from build123d import *

# Parameters (mm, degrees)
SKETCH1_R           = 11.495405
BOSS_EXTRUDE2_DEPTH = 4.7625
BOSS_EXTRUDE3_DEPTH = 3.175
FILLET1_R           = 1.5875


with BuildPart() as part:
    # Sketch1 → Boss-Extrude2 (new body, symmetric)
    with BuildSketch(Plane.XY):
        with BuildLine():
            ThreePointArc((14.672983865, 0.491098707), (-4.158599684, 14.079903484), (-12.585193267, -7.559797873))
            ThreePointArc((-12.585193267, -7.559797873), (4.158599684, -14.079903484), (14.672983865, 0.491098707))
        make_face()
        Circle(SKETCH1_R, mode=Mode.SUBTRACT)
    extrude(amount=BOSS_EXTRUDE2_DEPTH, both=True)

    # Sketch1<4> → Boss-Extrude3 (add, symmetric)
    with BuildSketch(Plane.XY):
        with BuildLine():
            ThreePointArc((-12.585193267, -7.559797873), (-10.89585042, -11.492870345), (-10.31875, -15.734319794))
            Line((-10.31875, -15.734319794), (-10.31875, -56.374319794))
            Line((-10.31875, -56.374319794), (8.54075, -56.374319794))
            Line((8.54075, -56.374319794), (8.54075, -76.694319794))
            Line((8.54075, -76.694319794), (34.499171822, -69.027315193))
            Line((34.499171822, -69.027315193), (23.458960581, -51.968120144))
            Line((23.458960581, -51.968120144), (39.292025986, -41.721424085))
            Line((39.292025986, -41.721424085), (17.211603503, -7.603033986))
            ThreePointArc((17.211603503, -7.603033986), (15.391641433, -3.728672569), (14.672983865, 0.491098707))
            ThreePointArc((14.672983865, 0.491098707), (4.158599684, -14.079903484), (-12.585193267, -7.559797873))
        make_face()
        with BuildLine():
            ThreePointArc((5.55625, -46.055569794), (0, -51.611819794), (-5.55625, -46.055569794))
            Line((-5.55625, -46.055569794), (-5.55625, -34.943069794))
            ThreePointArc((-5.55625, -34.943069794), (0, -29.386819794), (5.55625, -34.943069794))
            Line((5.55625, -34.943069794), (5.55625, -46.055569794))
        make_face(mode=Mode.SUBTRACT)
        with BuildLine():
            ThreePointArc((29.687419875, -35.646101109), (28.04160399, -43.329532516), (20.358172583, -41.683716631))
            Line((20.358172583, -41.683716631), (14.32055706, -32.354469339))
            ThreePointArc((14.32055706, -32.354469339), (15.966372945, -24.671037931), (23.649804353, -26.316853816))
            Line((23.649804353, -26.316853816), (29.687419875, -35.646101109))
        make_face(mode=Mode.SUBTRACT)
    extrude(amount=BOSS_EXTRUDE3_DEPTH, both=True)

    # Fillet1
    fillet1_edges = [part.edges().sort_by_distance(p)[0] for p in [
        (34.499171822, -69.027315193, 0),
        (23.458960581, -51.968120144, 0),
        (39.292025986, -41.721424085, 0),
        (-10.31875, -56.374319794, 0),
        (8.54075, -56.374319794, 0),
        (8.54075, -76.694319794, 0),
    ]]
    fillet(fillet1_edges, radius=FILLET1_R)


solid = part.part
Here's how the part is built. I have some questions about the finished solid (model axes, mm). A direction names the side the tool comes from. Coordinates: 2 decimals unless noted, no trailing zeros. Loops run counter-clockwise (first coordinate to the right, second up) from the corner with the lowest first, then second, coordinate; pieces in that order, holes last. Notation, with made-up numbers: (-0.5, 65) -> (41.5, 65) arc R23 ccw to (41.5, 90) -> close; hole circle Ø9 at (-9, -24). An arc over 180 degrees is marked (long way). Use one line per item in the form item = value. Start each with the question number.
(1) Please list where these lines run through material, in increasing order: line 1 along Y through (x, z) = (0, 1.9); line 2 along Y through (x, z) = (0, 3.4); line 3 along X through (y, z) = (-31, 1.25).
(2) On a 3-axis mill with a long thin cutter (end or side, diameter ignored), from which of +Z, -Z, +X, -X, +Y, -Y can I reach the whole of each face in a straight line? I mean faces 1 (the face through (-1, -56.374, 0)), 2 (the face through (28.896, -60.37, 0.044)), 3 (the face through (26.63, -30.92, 0.04)). Say none if no direction works.
(3) If we section it at C-C (y = -47.5): Please give me the cut outline in (x, z) (3 decimals), then the cut area to 3 significant figures.
(4) If we section it at A-A (x = 0): Please give me the cut outline in (y, z) (1 decimal).
(5) If we section it at D-D (x = 26): Please give me the cut outline in (y, z) (1 decimal), then the cut area to 3 significant figures.
(6) If we section it at B-B (z = 1.75): Give the number of separate pieces and of enclosed holes in the cut face, then the cut area to 3 significant figures.
(7) Will these pins go through, and if not, where does the flat tip stop? pin 1 (3 mm diameter, centred on x = -5, z = 1.5, fed in from -Y); pin 2 (4 mm diameter, centred on y = -24, z = 3.5, fed in from +X); pin 3 (1.9 mm diameter, centred on y = -35.5, z = 1, fed in from -X); pin 4 (18.5 mm diameter, centred on x = 0, y = 0, fed in from +Z).
Verdict:
q1.line_1 = -56.37 to -51.61, -29.39 to -11.5, 11.5 to 14.68
q1.line_2 = -14.68 to -11.5, 11.5 to 14.68
q1.line_3 = -10.32 to -3.91, 3.91 to 13.68, 26.68 to 32.35
q2.face_1 = +Z, -Z, -X, -Y
q2.face_2 = +Z, -Z, +X
q2.face_3 = +Z, -Z
q3.outline = (-10.319, -3.175) -> (-5.365, -3.175) -> (-5.365, 3.175) -> (-10.319, 3.175) -> close; (5.365, -3.175) -> (30.363, -3.175) -> (30.363, 3.175) -> (5.365, 3.175) -> close
q3.area = 190 mm²
q4.outline = (-56.4, -3.2) -> (-51.6, -3.2) -> (-51.6, 3.2) -> (-56.4, 3.2) -> close; (-29.4, -3.2) -> (-14.7, -3.2) -> (-14.7, -4.8) -> (-11.5, -4.8) -> (-11.5, 4.8) -> (-14.7, 4.8) -> (-14.7, 3.2) -> (-29.4, 3.2) -> close; (11.5, -4.8) -> (14.7, -4.8) -> (14.7, 4.8) -> (11.5, 4.8) -> close
q5.outline = (-71.5, -3.2) -> (-55.9, -3.2) -> (-55.9, 3.2) -> (-71.5, 3.2) -> close; (-50.3, -3.2) -> (-44.1, -3.2) -> (-44.1, 3.2) -> (-50.3, 3.2) -> close; (-29.9, -3.2) -> (-21.2, -3.2) -> (-21.2, 3.2) -> (-29.9, 3.2) -> close
q5.area = 194 mm²
q6.separate_pieces = 1
q6.enclosed_holes = 3
q6.area = 1,990 mm²
q7.pin_1 = -56.37
q7.pin_2 = 29.1
q7.pin_3 = -10.32
q7.pin_4 = through
